```python
from build123d import *

# Parameters (mm, degrees)
SKETCH1_W           = 50
SKETCH1_H           = 86.65
BOSS_EXTRUDE1_DEPTH = 7.5
SKETCH7_W           = 5.5
SKETCH7_H           = 62.4
CUT_EXTRUDE5_DEPTH  = 5.95
SKETCH11_R          = 2.1
CUT_EXTRUDE8_DEPTH  = 8.5
SKETCH12_R          = 2.1
CUT_EXTRUDE10_DEPTH = 8.5
SKETCH13_W          = 86.65
SKETCH13_H          = 7.5
BOSS_EXTRUDE2_DEPTH = 1
SKETCH14_W          = 86.65
SKETCH14_H          = 7.5
CUT_EXTRUDE11_DEPTH = 12


with BuildPart() as part:
    # Sketch1 → Boss-Extrude1 (new body)
    with BuildSketch(Plane(origin=(0, 0, 0), x_dir=(1, 0, 0), z_dir=(0, 1, 0))):
        Rectangle(SKETCH1_W, SKETCH1_H)
    extrude(amount=BOSS_EXTRUDE1_DEPTH)

    # Sketch7 → Cut-Extrude5 (cut)
    with BuildSketch(Plane(origin=(0, 7.5, 0), x_dir=(1, 0, 0), z_dir=(0, 1, 0))):
        with Locations((-8.15, -3.875)):
            Rectangle(SKETCH7_W, SKETCH7_H)
    extrude(amount=-CUT_EXTRUDE5_DEPTH, mode=Mode.SUBTRACT)

    # Sketch11 → Cut-Extrude8 (cut, through all)
    with BuildSketch(Plane(origin=(0, 7.5, 0), x_dir=(1, 0, 0), z_dir=(0, 1, 0))):
        with Locations((15.982, 35.325)):
            Circle(SKETCH11_R)
        with Locations((-8.018, 35.325)):
            Circle(SKETCH11_R)
    extrude(amount=-CUT_EXTRUDE8_DEPTH, mode=Mode.SUBTRACT)

    # Sketch12 → Cut-Extrude10 (cut, through all)
    with BuildSketch(Plane(origin=(0, 7.5, 0), x_dir=(1, 0, 0), z_dir=(0, 1, 0))):
        with Locations((20.25, 10.821)):
            Circle(SKETCH12_R)
        with Locations((20.25, -38.229)):
            Circle(SKETCH12_R)
    extrude(amount=-CUT_EXTRUDE10_DEPTH, mode=Mode.SUBTRACT)

    # Sketch13 → Boss-Extrude2 (add)
    with BuildSketch(Plane(origin=(25, 0, 0), x_dir=(0, 0, -1), z_dir=(1, 0, 0))):
        with Locations((0, 3.75)):
            Rectangle(SKETCH13_W, SKETCH13_H)
    extrude(amount=BOSS_EXTRUDE2_DEPTH)

    # Sketch14 → Cut-Extrude11 (cut)
    with BuildSketch(Plane.ZY.offset(25)):
        with Locations((0, 3.75)):
            Rectangle(SKETCH14_W, SKETCH14_H)
    extrude(amount=-CUT_EXTRUDE11_DEPTH, mode=Mode.SUBTRACT)


solid = part.part
```
The listing builds one solid part. Answer for the finished solid, in the listing's coordinates (mm). A direction names the side the tool comes from. Give positions to 0.01 mm unless a question says otherwise; leave off trailing zeros. Order: outer loops, then holes, each group sorted by start corner. A loop starts at its lowest first (then second) coordinate and runs counter-clockwise, first axis right, second up. Notation, with made-up numbers: (47.25, -31) - (101.25, -31) arc R22 ccw to (101.25, -14) - close; hole circle Ø1 at (42, -30.75). An arc over 180 degrees is marked (long way). Use one line per item in the form item = value. Start each with the question number.
(1) The mould has two halves that part along Z. Classify faces 3 (the flat face through (6, 4, 43.325)), 4 (the flat face through (-10.9, 5, 4)), 5 (the flat face through (26, 4, 1)): released by +Z, released by -Z, zero draft, split by the parting line, or undercut.
(2) Flat-ended cylindrical pins translate along their axes: pin 1 Ø4 at (x, z) = (15.982, -35.325) entering from +Y; pin 2 Ø1.6 at (x, z) = (-8, -7) entering from +Y. Find the tip coordinate at first contact, or state that the pin passes through.
(3) For faces 1 (the flat face through (6, 0, 1)), 2 (the flat face through (-8, 5, -27.325)), determine the directions among +Z, -Z, +X, -X, +Y, -Y from which every point of the face is accessible in a straight line to the end or side of a thin tool.
(4) Consider line 1 (Z direction, x = 20.25, y = 5.25) (3 decimals); line 2 (X direction, y = 2.75, z = 21.5); line 3 (X direction, y = 0.75, z = -36). Determine where each line is inside the solid, lowest interval first. Write a range as from..to.
(5) A cutting plane is placed at D-D, the plane z = -34.5. Write down the section's boundary in (x, y).
(6) A cutting plane is placed at B-B, the plane z = 3.5. Write down the section's boundary in (x, y).
(7) A cutting plane is placed at A-A, the plane x = 20.25. Write down the section's boundary in (y, z) (3 decimals), then the cut area to 3 significant figures.
(8) A cutting plane is placed at C-C, the plane z = -9.5. Write down the section's boundary in (x, y).
Ans:
q1.face_3 = released by +Z
q1.face_4 = undercut
q1.face_5 = zero draft
q2.pin_1 = through
q2.pin_2 = 1.55
q3.face_1 = +Z, -Z, +X, -X, -Y
q3.face_2 = +Y
q4.line_1 = -43.325..-12.921, -8.721..36.129, 40.329..43.325
q4.line_2 = -13..-10.9, -5.4..26
q4.line_3 = -13..-10.01, -6.03..13.99, 17.97..26
q5.outline = (-13, 0) - (-9.95, 0) - (-9.95, 7.5) - (-13, 7.5) - close; (-6.09, 0) - (14.05, 0) - (14.05, 7.5) - (-6.09, 7.5) - close; (17.91, 0) - (26, 0) - (26, 7.5) - (17.91, 7.5) - close
q6.outline = (-13, 0) - (26, 0) - (26, 7.5) - (-5.4, 7.5) - (-5.4, 1.55) - (-10.9, 1.55) - (-10.9, 7.5) - (-13, 7.5) - close
q7.outline = (0, -43.325) - (7.5, -43.325) - (7.5, -12.921) - (0, -12.921) - close; (0, -8.721) - (7.5, -8.721) - (7.5, 36.129) - (0, 36.129) - close; (0, 40.329) - (7.5, 40.329) - (7.5, 43.325) - (0, 43.325) - close
q7.area = 587 mm^2
q8.outline = (-13, 0) - (18.62, 0) - (18.62, 7.5) - (-5.4, 7.5) - (-5.4, 1.55) - (-10.9, 1.55) - (-10.9, 7.5) - (-13, 7.5) - close; (21.88, 0) - (26, 0) - (26, 7.5) - (21.88, 7.5) - close
